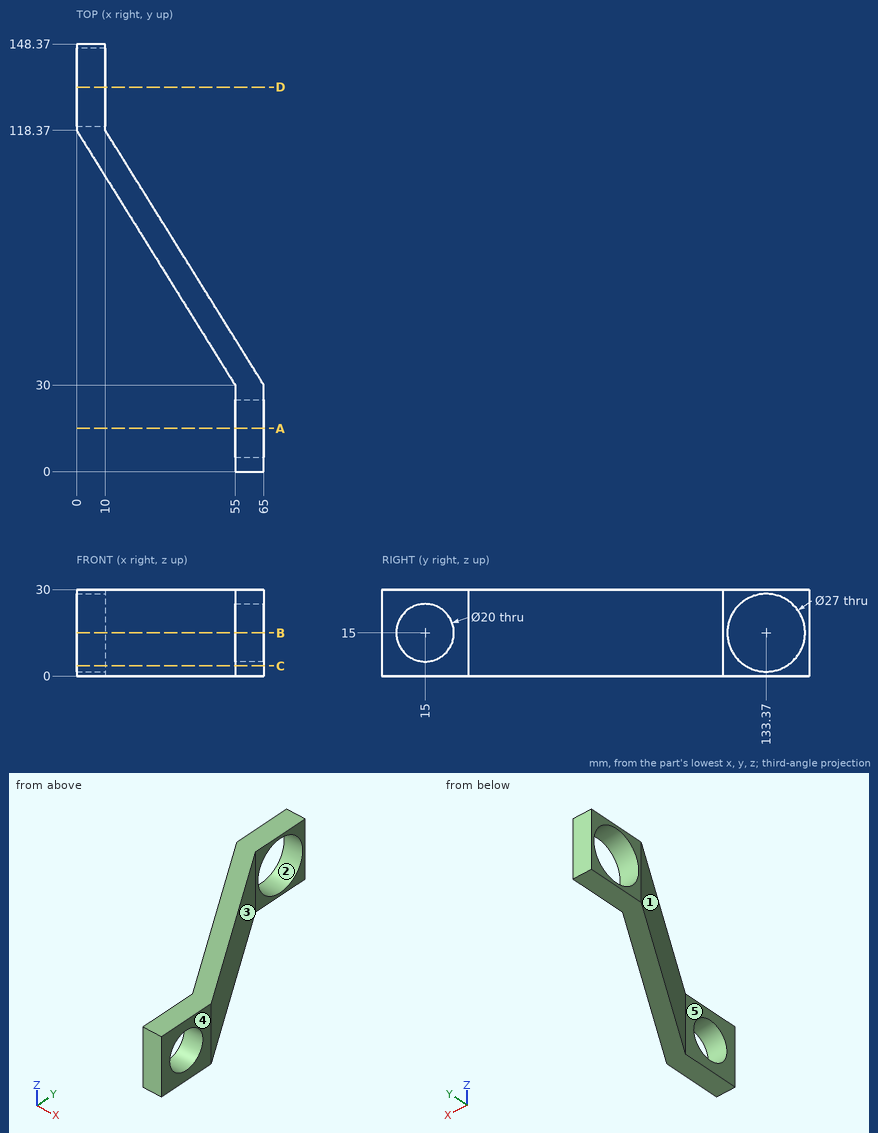
Could you check a few things on this drawing? It's one solid part, dimensions in mm from its lowest x, y, z. A direction names the side the tool comes from. Coordinates: 2 decimals unless noted, no trailing zeros. Order: outer loops, then holes, each group sorted by start corner. A loop starts at its lowest first (then second) coordinate and runs counter-clockwise, first axis right, second up.
1. If we section it at A-A (y = 15): Please give me the cut outline in (x, z).
2. For the marked faces 4 and 5, which set-ups out of +Z, -Z, +X, -X, +Y, -Y let a thin tool reach every point of the face, with its end or its side?
3. I need wall thicknesses on line 1 (Z direction, x = 4, y = 133); line 2 (Y direction, x = 56, z = 7.5); line 3 (X direction, y = 120.5, z = 24.25). Which ranges of each line are inside material? Lowest first, please.
4. If we section it at B-B (z = 15): Please give me the cut outline in (x, y).
5. If we section it at C-C (z = 3.5): Please give me the cut outline in (x, y), then the cut area to 3 significant figures.
6. If we section it at D-D (y = 133.37): Please give me the cut outline in (x, z).
7. Thinking about a two-plate mould opening in Y: for the marked faces 1, 2 and 3, which applies, +Y half, -Y half, draft (parallel to the pull), parting line (faces both ways), or undercut?
8. I'm going to push flat-ended pins straight in: pin 1 (10 mm diameter, centred on y = 50, z = 23.5, fed in from +X); pin 2 (18 mm diameter, centred on y = 15, z = 15, fed in from -X); pin 3 (8 mm diameter, centred on x = 38.5, z = 10, fed in from -Y). Where does each tip first touch, or does it pass through?
Entries:
1. outline: (55, 0) - (65, 0) - (65, 5) - (55, 5) - close; (55, 25) - (65, 25) - (65, 30) - (55, 30) - close
2. face 4: +Z, -Z, +X, +Y, -Y
2. face 5: +Z, -Z, -X, -Y
3. line 1: z = 0 to 1.51, 28.49 to 30
3. line 2: y = 0 to 8.39, 21.61 to 44.46
3. line 3: x = 0 to 10
4. outline: (0, 118.37) - (55, 30) - (55, 25) - (65, 25) - (65, 30) - (10, 118.37) - (10, 119.87) - (0, 119.87) - close; (0, 146.87) - (10, 146.87) - (10, 148.37) - (0, 148.37) - close; (55, 0) - (65, 0) - (65, 5) - (55, 5) - close
5. outline: (0, 118.37) - (55, 30) - (55, 0) - (65, 0) - (65, 30) - (10, 118.37) - (10, 126.3) - (0, 126.3) - close; (0, 140.44) - (10, 140.44) - (10, 148.37) - (0, 148.37) - close
5. area: 1,340 mm2
6. outline: (0, 0) - (10, 0) - (10, 1.5) - (0, 1.5) - close; (0, 28.5) - (10, 28.5) - (10, 30) - (0, 30) - close
7. face 1: -Y half
7. face 2: undercut
7. face 3: +Y half
8. pin 1: stops at x = 55.66
8. pin 2: passes through
8. pin 3: stops at y = 50.08
